Can you work these out from the model? Positions are in its coordinate system, mm. Round coordinates to 2 decimals unless told otherwise and drop trailing zeros. Order: outer loops, then holes, each group sorted by start corner. A loop starts at its lowest first (then second) coordinate and runs counter-clockwise, first axis right, second up. Notation, with made-up numbers: (-29.5, -28.75) -> (-23.5, -28.75) arc R9 cw to (-23.5, -20.75) -> close; hole circle Ø4 at (-36, 32). An arc over 180 degrees is marked (long way). One line per item, written item: value.
```python
from build123d import *

# Parameters (mm, degrees)
F1_DEPTH = 279.4
F2_W     = 508
F2_H     = 426.719844
F2_H_2   = 111.069546
F3_DEPTH = 304.8
F4_W     = 19.05
F4_H     = 50.8
F5_DEPTH = 12.7


with BuildPart() as f1:
    # F0 (on Top) → F1 (new body)
    with BuildSketch(Plane.XY):
        with BuildLine():
            Line((458.216, -9.525), (533.4, -9.525))
            Line((533.4, -9.525), (533.4, 9.525))
            Line((533.4, 9.525), (-533.4, 9.525))
            Line((-533.4, 9.525), (-533.4, -9.525))
            Line((-533.4, -9.525), (-509.016, -9.525))
            ThreePointArc((-509.016, -9.525), (-508.29758, -9.22742), (-508, -8.509))
            ThreePointArc((-508, -8.509), (-507.70242, -9.22742), (-506.984, -9.525))
            Line((-506.984, -9.525), (-458.216, -9.525))
            ThreePointArc((-458.216, -9.525), (-457.49758, -9.22742), (-457.2, -8.509))
            ThreePointArc((-457.2, -8.509), (-456.90242, -9.22742), (-456.184, -9.525))
            Line((-456.184, -9.525), (-407.416, -9.525))
            ThreePointArc((-407.416, -9.525), (-406.69758, -9.22742), (-406.4, -8.509))
            ThreePointArc((-406.4, -8.509), (-406.10242, -9.22742), (-405.384, -9.525))
            Line((-405.384, -9.525), (-356.616, -9.525))
            ThreePointArc((-356.616, -9.525), (-355.89758, -9.22742), (-355.6, -8.509))
            ThreePointArc((-355.6, -8.509), (-355.30242, -9.22742), (-354.584, -9.525))
            Line((-354.584, -9.525), (-305.816, -9.525))
            ThreePointArc((-305.816, -9.525), (-305.09758, -9.22742), (-304.8, -8.509))
            ThreePointArc((-304.8, -8.509), (-304.50242, -9.22742), (-303.784, -9.525))
            Line((-303.784, -9.525), (-255.016, -9.525))
            ThreePointArc((-255.016, -9.525), (-254.29758, -9.22742), (-254, -8.509))
            ThreePointArc((-254, -8.509), (-253.70242, -9.22742), (-252.984, -9.525))
            Line((-252.984, -9.525), (-204.216, -9.525))
            ThreePointArc((-204.216, -9.525), (-203.49758, -9.22742), (-203.2, -8.509))
            ThreePointArc((-203.2, -8.509), (-202.90242, -9.22742), (-202.184, -9.525))
            Line((-202.184, -9.525), (-153.416, -9.525))
            ThreePointArc((-153.416, -9.525), (-152.69758, -9.22742), (-152.4, -8.509))
            ThreePointArc((-152.4, -8.509), (-152.10242, -9.22742), (-151.384, -9.525))
            Line((-151.384, -9.525), (-102.616, -9.525))
            ThreePointArc((-102.616, -9.525), (-101.89758, -9.22742), (-101.6, -8.509))
            ThreePointArc((-101.6, -8.509), (-101.30242, -9.22742), (-100.584, -9.525))
            Line((-100.584, -9.525), (-51.816, -9.525))
            ThreePointArc((-51.816, -9.525), (-51.09758, -9.22742), (-50.8, -8.509))
            ThreePointArc((-50.8, -8.509), (-50.50242, -9.22742), (-49.784, -9.525))
            Line((-49.784, -9.525), (-1.016, -9.525))
            ThreePointArc((-1.016, -9.525), (-0.29758, -9.22742), (0, -8.509))
            ThreePointArc((0, -8.509), (0.29758, -9.22742), (1.016, -9.525))
            Line((1.016, -9.525), (49.784, -9.525))
            ThreePointArc((49.784, -9.525), (50.50242, -9.22742), (50.8, -8.509))
            ThreePointArc((50.8, -8.509), (51.09758, -9.22742), (51.816, -9.525))
            Line((51.816, -9.525), (100.584, -9.525))
            ThreePointArc((100.584, -9.525), (101.30242, -9.22742), (101.6, -8.509))
            ThreePointArc((101.6, -8.509), (101.89758, -9.22742), (102.616, -9.525))
            Line((102.616, -9.525), (151.384, -9.525))
            ThreePointArc((151.384, -9.525), (152.10242, -9.22742), (152.4, -8.509))
            ThreePointArc((152.4, -8.509), (152.69758, -9.22742), (153.416, -9.525))
            Line((153.416, -9.525), (202.184, -9.525))
            ThreePointArc((202.184, -9.525), (202.90242, -9.22742), (203.2, -8.509))
            ThreePointArc((203.2, -8.509), (203.49758, -9.22742), (204.216, -9.525))
            Line((204.216, -9.525), (252.984, -9.525))
            ThreePointArc((252.984, -9.525), (253.70242, -9.22742), (254, -8.509))
            ThreePointArc((254, -8.509), (254.29758, -9.22742), (255.016, -9.525))
            Line((255.016, -9.525), (303.784, -9.525))
            ThreePointArc((303.784, -9.525), (304.50242, -9.22742), (304.8, -8.509))
            ThreePointArc((304.8, -8.509), (305.09758, -9.22742), (305.816, -9.525))
            Line((305.816, -9.525), (354.584, -9.525))
            ThreePointArc((354.584, -9.525), (355.30242, -9.22742), (355.6, -8.509))
            ThreePointArc((355.6, -8.509), (355.89758, -9.22742), (356.616, -9.525))
            Line((356.616, -9.525), (405.384, -9.525))
            ThreePointArc((405.384, -9.525), (406.10242, -9.22742), (406.4, -8.509))
            ThreePointArc((406.4, -8.509), (406.69758, -9.22742), (407.416, -9.525))
            Line((407.416, -9.525), (456.184, -9.525))
            ThreePointArc((456.184, -9.525), (456.90242, -9.22742), (457.2, -8.509))
            ThreePointArc((457.2, -8.509), (457.49758, -9.22742), (458.216, -9.525))
        make_face()
        with BuildLine():
            ThreePointArc((-508, -8.509), (-508.29758, -9.22742), (-509.016, -9.525))
            Line((-509.016, -9.525), (-506.984, -9.525))
            ThreePointArc((-506.984, -9.525), (-507.70242, -9.22742), (-508, -8.509))
        make_face()
    extrude(amount=F1_DEPTH)

    # F2 (on Top) → F3 (cut, symmetric)
    with BuildSketch(Plane.XY):
        with Locations((-406.4, 0)):
            Rectangle(F2_W, F2_H)
        with Locations((406.4, 0)):
            Rectangle(F2_W, F2_H_2)
    extrude(amount=F3_DEPTH, both=True, mode=Mode.SUBTRACT)

    # F4 (on Front) → F5 (cut, symmetric)
    with BuildSketch(Plane.XZ):
        with Locations((142.875, 254)):
            Rectangle(F4_W, F4_H)
        with Locations((-142.875, 254)):
            Rectangle(F4_W, F4_H)
    extrude(amount=F5_DEPTH, both=True, mode=Mode.SUBTRACT)


solid = f1.part
```
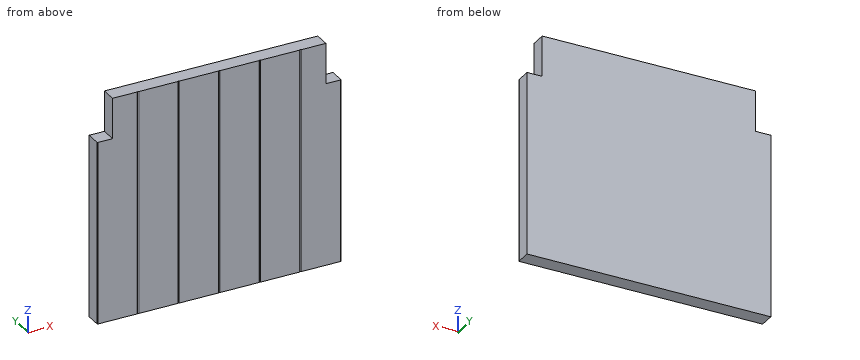
Q1. I want a section at B-B on z = 234. List the corners of the cut face in (x, y) for me (3 decimals), plus the area to 3 significant figures.
Answers below:
outline: (-133.35, -9.525) -> (-102.616, -9.525) arc R1.016 ccw to (-101.6, -8.509) arc R1.016 ccw to (-100.584, -9.525) -> (-51.816, -9.525) arc R1.016 ccw to (-50.8, -8.509) arc R1.016 ccw to (-49.784, -9.525) -> (-1.016, -9.525) arc R1.016 ccw to (0, -8.509) arc R1.016 ccw to (1.016, -9.525) -> (49.784, -9.525) arc R1.016 ccw to (50.8, -8.509) arc R1.016 ccw to (51.816, -9.525) -> (100.584, -9.525) arc R1.016 ccw to (101.6, -8.509) arc R1.016 ccw to (102.616, -9.525) -> (133.35, -9.525) -> (133.35, 9.525) -> (-133.35, 9.525) -> close
area: 5,080 mm^2
Q2. Will these pins go through, and if not, where does the flat tip stop? pin 1 Ø5.5 at (y, z) = (1.5, 266) entering from -X; pin 2 Ø5.5 at (y, z) = (4.5, 246.5) entering from +X.
Answers below:
pin 1: x = -133.35
pin 2: x = 133.35
Q3. I want a section at A-A on y = 6. List the corners of the cut face in (x, z) for me, plus the area to 3 significant figures.
Answers below:
outline: (-152.4, 0) -> (152.4, 0) -> (152.4, 228.6) -> (133.35, 228.6) -> (133.35, 279.4) -> (-133.35, 279.4) -> (-133.35, 228.6) -> (-152.4, 228.6) -> close
area: 83,200 mm^2
Q4. Please list where these lines run through material, in increasing order: line 1 along X through (y, z) = (-5, 248); line 2 along Y through (x, z) = (101, 54) (3 decimals).
Answers below:
line 1: -133.35 to 133.35
line 2: -9.436 to 9.525
